The drawing under review shows one solid part. Ordinate dimensions are in mm from its lowest x, y, z. Coordinates: 2 decimals unless noted, no trailing zeros. Order: outer loops, then holes, each group sorted by start corner. A loop starts at its lowest first (then second) coordinate and runs counter-clockwise, first axis right, second up.
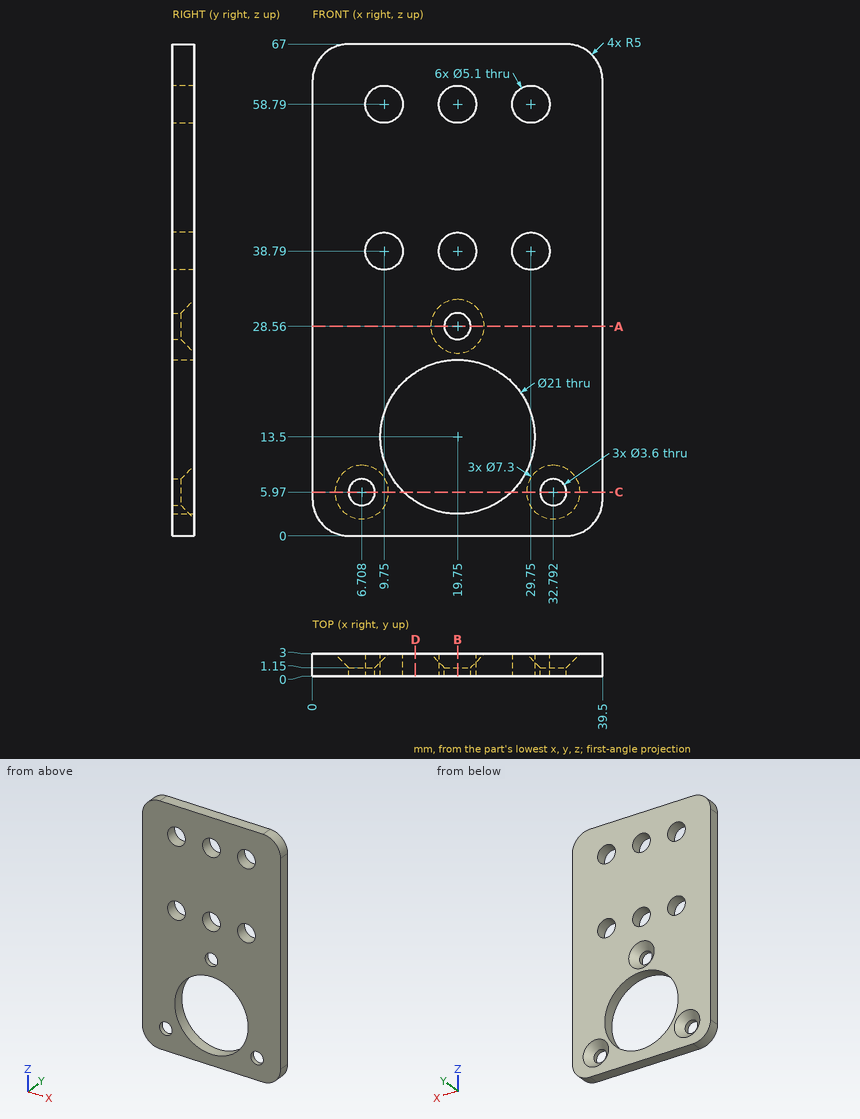
(1) For pin 1 Ø8 at (x, z) = (29.75, 58.79) entering from +Y, flat-tipped, find the tip position at first contact; note if it passes through.
A:
pin 1: stops at y = 3
(2) Wall thickness on probe 1 along Z at (x, y) = (19.75, 0.7); probe 2 along X at (y, z) = (1.5, 59); probe 3 along X at (y, z) = (0.6, 5.97): over which ranges is each line inside the solid? List them lowest first.
A:
probe 1: z = 0 to 3, 24 to 26.76, 30.36 to 36.24, 41.34 to 56.24, 61.34 to 67
probe 2: x = 0 to 7.21, 12.29 to 17.21, 22.29 to 27.21, 32.29 to 39.5
probe 3: x = 0 to 4.91, 8.51 to 12.43, 27.07 to 30.99, 34.59 to 39.5
(3) We need section C-C, the plane z = 5.97. Write out the cut boundary in (x, y).
A:
outline: (0, 0) - (4.91, 0) - (4.91, 1.15) - (3.06, 3) - (0, 3) - close; (8.51, 0) - (12.43, 0) - (12.43, 3) - (10.36, 3) - (8.51, 1.15) - close; (27.07, 0) - (30.99, 0) - (30.99, 1.15) - (29.14, 3) - (27.07, 3) - close; (34.59, 0) - (39.5, 0) - (39.5, 3) - (36.44, 3) - (34.59, 1.15) - close
(4) We need section A-A, the plane z = 28.56. Write out the cut boundary in (x, y), and give its area (3 significant figures).
A:
outline: (0, 0) - (17.95, 0) - (17.95, 1.15) - (16.1, 3) - (0, 3) - close; (21.55, 0) - (39.5, 0) - (39.5, 3) - (23.4, 3) - (21.55, 1.15) - close
area: 104 mm2
(5) We need section D-D, the plane x = 14. Write out the cut boundary in (y, z) (1 decimal), and give its area (3 significant figures).
A:
outline: (0, 0) - (3, 0) - (3, 4.7) - (0, 4.7) - close; (0, 22.3) - (3, 22.3) - (3, 67) - (0, 67) - close
area: 148 mm2
(6) We need section B-B, the plane x = 19.75. Write out the cut boundary in (y, z).
A:
outline: (0, 0) - (3, 0) - (3, 3) - (0, 3) - close; (0, 24) - (3, 24) - (3, 24.91) - (1.15, 26.76) - (0, 26.76) - close; (0, 30.36) - (1.15, 30.36) - (3, 32.21) - (3, 36.24) - (0, 36.24) - close; (0, 41.34) - (3, 41.34) - (3, 56.24) - (0, 56.24) - close; (0, 61.34) - (3, 61.34) - (3, 67) - (0, 67) - close
